Geometry: final body of the model. Coordinates: model frame, mm. Face numbers are marked on the shaded views. A direction names the side the tool comes from. Give positions to 0.01 mm unless a question says otherwise; leave off trailing zeros. Loops run counter-clockwise (first coordinate to the right, second up) from the corner with the lowest first, then second, coordinate; pieces in that order, holes last. Notation, with made-up numbers: M 86,-28.75 L 145,-28.75 A9 ccw 145,-15.75 Z; hole C 14.5,59.5 d8. An arc over 180 degrees is marked long. One line per question, with ' | ' between items. Start each with the question number.
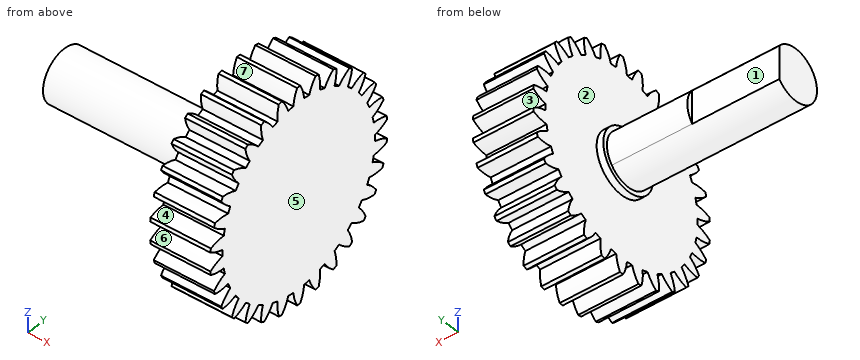
from build123d import *

# Parameters (mm, degrees)
BASPROSKE_W              = 9
BASPROSKE_H              = 16
TOOTHCUT_DEPTH           = 25.351591324
TEETHCUTS_COUNT          = 30
TEETHCUTS_ANGLE          = 348
BORSKE_R                 = 4
BORE_DEPTH               = 50.0000508
BOSS_EXTRUDE3_DEPTH      = 26
BOSS_EXTRUDE3_DEPTH_BACK = 9
BOSS_EXTRUDE4_DEPTH      = 13
BOSS_EXTRUDE4_DEPTH_BACK = 9
SKETCH2_6_R              = 4.5
SKETCH2_6_R_2            = 3.85
BOSS_EXTRUDE5_DEPTH      = 1
BOSS_EXTRUDE5_DEPTH_BACK = 9


with BuildPart() as part:
    # BasProSke → Base-Revolve (revolve)
    with BuildSketch(Plane(origin=(0, 0, 0), x_dir=(1, 0, 0), z_dir=(0, 1, 0)), mode=Mode.PRIVATE) as base_revolve_sk:
        with Locations((4.5, 8)):
            Rectangle(BASPROSKE_W, BASPROSKE_H)
    revolve(base_revolve_sk.sketch.rotate(Axis((-10, 0, 0), (1, 0, 0)), 180), axis=Axis((-10, 0, 0), (1, 0, 0)))

    # TooCutSke → ToothCut (cut, through all)
    with BuildSketch(Plane(origin=(0, 0, 0), x_dir=(0, 0, -1), z_dir=(1, 0, 0))):
        with BuildLine():
            ThreePointArc((0.466400716, 13.741086979), (0, 13.749), (-0.466400716, 13.741086979))
            ThreePointArc((-0.466400716, 13.741086979), (-0.819142092, 14.899954875), (-1.3974676, 15.964351834))
            ThreePointArc((-1.3974676, 15.964351834), (0, 16.0254), (1.3974676, 15.964351834))
            ThreePointArc((1.3974676, 15.964351834), (0.819142092, 14.899954875), (0.466400716, 13.741086979))
        make_face()
    toothcut = extrude(amount=TOOTHCUT_DEPTH, mode=Mode.SUBTRACT)

    # TeethCuts: ToothCut ×30 about axis
    teethcuts_axis = Axis((-10, 0, 0), (1, 0, 0))
    for i in range(1, TEETHCUTS_COUNT):
        add(toothcut.rotate(teethcuts_axis, i * TEETHCUTS_ANGLE / (TEETHCUTS_COUNT - 1)), mode=Mode.SUBTRACT)

    # BorSke → Bore (cut, symmetric)
    with BuildSketch(Plane(origin=(0, 0, 0), x_dir=(0, 0, -1), z_dir=(1, 0, 0))):
        with Locations(Location((0, 0, 0), (0, 0, 180))):
            Circle(BORSKE_R)
    extrude(amount=BORE_DEPTH, both=True, mode=Mode.SUBTRACT)



with BuildPart() as body_2:
    # Sketch2 → Boss-Extrude3 (new, two sides)
    with BuildSketch(Plane.ZY) as boss_extrude3_sk:
        with BuildLine():
            Line((2.45, 2.969848481), (-2.45, 2.969848481))
            ThreePointArc((-2.45, 2.969848481), (-1.641645516, -3.48245603), (3.85, 0))
            ThreePointArc((3.85, 0), (3.48245603, 1.641645516), (2.45, 2.969848481))
        make_face()
    extrude(amount=BOSS_EXTRUDE3_DEPTH)
    extrude(boss_extrude3_sk.sketch, amount=-BOSS_EXTRUDE3_DEPTH_BACK)

    # Sketch2_5 → Boss-Extrude4 (add, two sides)
    with BuildSketch(Plane.ZY) as boss_extrude4_sk:
        with BuildLine():
            ThreePointArc((2.45, 2.969848481), (0, 3.85), (-2.45, 2.969848481))
            Line((-2.45, 2.969848481), (2.45, 2.969848481))
        make_face()
        with BuildLine():
            Line((2.45, 2.969848481), (-2.45, 2.969848481))
            ThreePointArc((-2.45, 2.969848481), (-1.641645516, -3.48245603), (3.85, 0))
            ThreePointArc((3.85, 0), (3.48245603, 1.641645516), (2.45, 2.969848481))
        make_face()
    extrude(amount=BOSS_EXTRUDE4_DEPTH)
    extrude(boss_extrude4_sk.sketch, amount=-BOSS_EXTRUDE4_DEPTH_BACK)


with BuildPart() as part_1:
    add(part.part)

    add(body_2.part)  # Boss-Extrude5 merges body 2
    # Sketch2_6 → Boss-Extrude5 (add, two sides)
    with BuildSketch(Plane.ZY) as boss_extrude5_sk:
        Circle(SKETCH2_6_R)
        Circle(SKETCH2_6_R_2, mode=Mode.SUBTRACT)
    extrude(amount=BOSS_EXTRUDE5_DEPTH)
    extrude(boss_extrude5_sk.sketch, amount=-BOSS_EXTRUDE5_DEPTH_BACK)


solid = part_1.part
Q1. Section B-B, the plane x = -9. Output: boundary loops of the cut face in (y, z).
Q2. Contact query for flat-ended pins moving along their axis: pin 1 (10 mm diameter, centred on x = -20, y = 1, fed in from -Z); pin 2 (4 mm diameter, centred on x = 0.5, y = -4, fed in from +Z); pin 3 (6 mm diameter, centred on y = -8.5, z = 0, fed in from -X). Output: stop coordinate, or through.
Q3. Section C-C, the plane x = -14. Output: boundary loops of the cut face in (y, z), plus the area to 3 significant figures.
Q4. Set-up query: the marked faces 1, 2 and 3. Return all of +Z, -Z, +X, -X, +Y, -Y with unobstructed straight access to the full face (end or side cutting, diameter ignored); none if empty.
Q5. Draft query along Z for the marked faces 4, 5, 6 and 7. Return one class per face: released by +Z, released by -Z, zero draft, split by the parting line, or undercut.
Q6. Material intervals for L1, parallel to Z at x = 5.5, y = 13; L2, parallel to Y at x = 5.5, z = 15.5; L3, parallel to Z at x = 2.5, y = -11, sorted ascending.
Q7. Section A-A, the plane z = 0. Output: boundary loops of the cut face in (x, y), plus the area to 3 significant figures.
Model answer:
1) outline: C 0,0 d7.7
2) pin 1: stops at z = -3.85 | pin 2: stops at z = 15.71 | pin 3: stops at x = 0
3) outline: M 2.97,-2.45 L 2.97,2.45 A3.85 ccw long Z | area: 43.6 mm^2
4) face 1: +Z, -Z, -X, +Y | face 2: -X | face 3: +X, -X, +Y
5) face 4: undercut | face 5: zero draft | face 6: undercut | face 7: released by +Z
6) L1: z = -8.19 to -6.53, -5.22 to 5.22, 6.53 to 8.19 | L2: y = -3.64 to -2.87, -0.53 to 0.53, 2.87 to 3.64 | L3: z = -10.7 to -8.63, -8.25 to 8.25, 8.63 to 10.7
7) outline: M -26,-3.85 L -1,-3.85 L -1,-4.5 L 0,-4.5 L 0,-13.75 L 9,-13.75 L 9,13.75 L 0,13.75 L 0,4.5 L -1,4.5 L -1,3.85 L -13,3.85 L -13,2.97 L -26,2.97 Z | area: 438 mm^2
